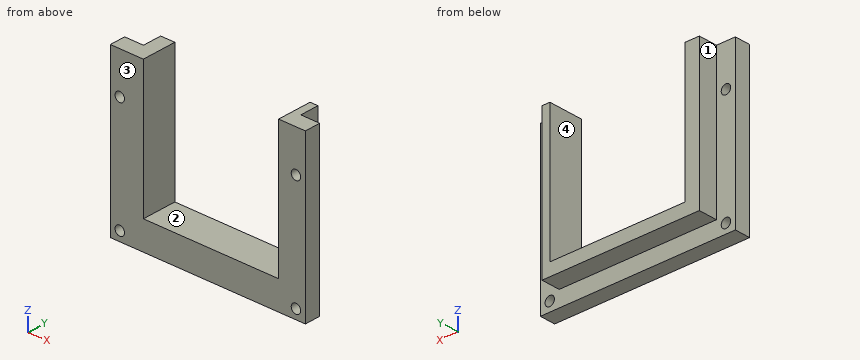
from build123d import *

# Parameters (mm, degrees)
IZIM1_R                     = 1.5
Y_KSEKLIK_EKSTR_ZYON1_DEPTH = 5
IZIM1_3_W                   = 50
IZIM1_3_H                   = 47
IZIM1_3_R                   = 2
Y_KSEKLIK_EKSTR_ZYON2_DEPTH = 11
IZIM4_W                     = 43
IZIM4_H                     = 43
IZIM4_R                     = 2
KES_EKSTR_ZYON9_DEPTH       = 20


with BuildPart() as part:
    # izim1 → Y_kseklik-Ekstr_zyon1 (new body)
    with BuildSketch(Plane(origin=(0, 0, 0), x_dir=(1, 0, 0), z_dir=(0, 1, 0))):
        Polygon((0, 52), (0, 0), (6, 0), (6, 47), (56, 47), (56, 0), (62, 0), (62, 52), align=None)
        with Locations(Location((3, 13, 0), (0, 0, 270))):
            Circle(IZIM1_R, mode=Mode.SUBTRACT)
        with Locations(Location((59, 13, 0), (0, 0, 270))):
            Circle(IZIM1_R, mode=Mode.SUBTRACT)
        with Locations(Location((3, 49, 0), (0, 0, 270))):
            Circle(IZIM1_R, mode=Mode.SUBTRACT)
        with Locations(Location((59, 49, 0), (0, 0, 270))):
            Circle(IZIM1_R, mode=Mode.SUBTRACT)
    extrude(amount=Y_KSEKLIK_EKSTR_ZYON1_DEPTH)

    # izim1_3 → Y_kseklik-Ekstr_zyon2 (add)
    with BuildSketch(Plane(origin=(0, 0, 0), x_dir=(1, 0, 0), z_dir=(0, 1, 0))):
        with Locations((31, 23.5)):
            Rectangle(IZIM1_3_W, IZIM1_3_H)
        with Locations(Location((16.5, 5.5, 0), (0, 0, 270))):
            Circle(IZIM1_3_R, mode=Mode.SUBTRACT)
        with Locations(Location((47.5, 5.5, 0), (0, 0, 270))):
            Circle(IZIM1_3_R, mode=Mode.SUBTRACT)
        with Locations(Location((16.5, 36.5, 0), (0, 0, 270))):
            Circle(IZIM1_3_R, mode=Mode.SUBTRACT)
        with Locations(Location((47.5, 36.5, 0), (0, 0, 270))):
            Circle(IZIM1_3_R, mode=Mode.SUBTRACT)
    extrude(amount=Y_KSEKLIK_EKSTR_ZYON2_DEPTH)

    # izim4 → Kes-Ekstr_zyon9 (cut)
    with BuildSketch(Plane(origin=(0, 0, 0), x_dir=(1, 0, 0), z_dir=(0, 1, 0))):
        with Locations((32, 21.5)):
            Rectangle(IZIM4_W, IZIM4_H)
        with Locations((16.5, 36.5)):
            Circle(IZIM4_R, mode=Mode.SUBTRACT)
        with Locations((47.5, 36.5)):
            Circle(IZIM4_R, mode=Mode.SUBTRACT)
        with Locations((47.5, 5.5)):
            Circle(IZIM4_R, mode=Mode.SUBTRACT)
        with Locations((16.5, 5.5)):
            Circle(IZIM4_R, mode=Mode.SUBTRACT)
    extrude(amount=KES_EKSTR_ZYON9_DEPTH, mode=Mode.SUBTRACT)


solid = part.part
Could you check a few things on this model? Use its own coordinates, in mm. Face numbers are marked on the shaded views. Round coordinates to 2 decimals unless told otherwise and drop trailing zeros. Write each loop counter-clockwise with the first axis right and the second up, starting at its lowest first coordinate (ties: lowest second). Pieces come first, ordered by that corner, then holes. Notation, with made-up numbers: (-11, -8) - (8, -8) arc R28 ccw to (8, 29) - close; hole circle Ø10 at (18, 24). An arc over 180 degrees is marked (long way). Use a Markdown table: item, result.
Q1. I want a section at B-B (z = -7.5). List the corners of the cut face in (x, y) for me, plus the area to 3 significant figures.
Output values:
| item | result |
|---|---|
| outline | (0, 0) - (10.5, 0) - (10.5, 11) - (6, 11) - (6, 5) - (0, 5) - close; (53.5, 0) - (62, 0) - (62, 5) - (56, 5) - (56, 11) - (53.5, 11) - close |
| area | 137 mm2 |
Q2. I want a section at C-C (y = 10). List the corners of the cut face in (x, z) for me.
Output values:
| item | result |
|---|---|
| outline | (6, -47) - (56, -47) - (56, 0) - (53.5, 0) - (53.5, -43) - (10.5, -43) - (10.5, 0) - (6, 0) - close |
Q3. I want a section at A-A (z = -49). List the corners of the cut face in (x, y) for me, plus the area to 3 significant figures.
Output values:
| item | result |
|---|---|
| outline | (0, 0) - (1.5, 0) - (1.5, 5) - (0, 5) - close; (4.5, 0) - (57.5, 0) - (57.5, 5) - (4.5, 5) - close; (60.5, 0) - (62, 0) - (62, 5) - (60.5, 5) - close |
| area | 280 mm2 |
Q4. I want a section at D-D (x = 3). List the corners of the cut face in (y, z) for me.
Output values:
| item | result |
|---|---|
| outline | (0, -52) - (5, -52) - (5, -50.5) - (0, -50.5) - close; (0, -47.5) - (5, -47.5) - (5, -14.5) - (0, -14.5) - close; (0, -11.5) - (5, -11.5) - (5, 0) - (0, 0) - close |
Q5. For pin 1 (1.8 mm diameter, centred on y = 7.5, z = -24.5, fed in from -X); pin 2 (5.5 mm diameter, centred on x = 29, y = 6.5, fed in from +Z); pin 3 (5 mm diameter, centred on x = 3, z = -49, fed in from +Y); pin 4 (2.5 mm diameter, centred on x = 59, z = -13, fed in from -Y), each with a flat end and sliding along its axis, tell me the tip position at first contact or that it passes through.
Output values:
| item | result |
|---|---|
| pin 1 | x = 6 |
| pin 2 | z = -43 |
| pin 3 | y = 5 |
| pin 4 | through |
Q6. Thinking about a two-plate mould opening in X: for the marked faces 1, 2, 3 and 4, which applies, released by +X, released by -X, zero draft, split by the parting line, or undercut?
Output values:
| item | result |
|---|---|
| face 1 | released by -X |
| face 2 | undercut |
| face 3 | zero draft |
| face 4 | undercut |
Q7. Please list where these lines run through material, in increasing order: L1, parallel to X at y = 1.35, z = -49; L2, parallel to X at y = 1.1, z = -13; L3, parallel to X at y = 7.75, z = -7.
Output values:
| item | result |
|---|---|
| L1 | 0 to 1.5, 4.5 to 57.5, 60.5 to 62 |
| L2 | 0 to 1.5, 4.5 to 10.5, 53.5 to 57.5, 60.5 to 62 |
| L3 | 6 to 10.5, 53.5 to 56 |
